Check sheet for the modelled part. Datum: model origin and axes. Units: mm. A direction names the side the tool comes from. Give positions to 0.01 mm unless a question says otherwise; leave off trailing zeros. Write each loop counter-clockwise with the first axis right and the second up, starting at its lowest first coordinate (ties: lowest second). Pieces come first, ordered by that corner, then holes. Notation, with made-up numbers: M 46,84 L 51,84 A23 cw 51,123 Z; hole C 29.5,-9 d2. An arc over 180 degrees is marked long. One line per item, written item: value. Start each with the question number.
from build123d import *

# Parameters (mm, degrees)
BOSS_EXTRUDE1_DEPTH        = 9
BOSS_EXTRUDE2_DEPTH        = 6
BOSS_EXTRUDE3_DEPTH        = 15
BOSS_EXTRUDE3_DEPTH_BACK   = 85
BOSS_EXTRUDE4_DEPTH        = 15
BOSS_EXTRUDE4_DEPTH_BACK   = 35
CUT_EXTRUDE1_DEPTH         = 10
CUT_EXTRUDE2_DEPTH         = 10
BOSS_EXTRUDE6_DEPTH        = 15
BOSS_EXTRUDE6_DEPTH_BACK   = 85
SKETCH1_6_R                = 25
F_25_0_25_DIAMETER_HOLE1_D = 25


with BuildPart() as part:
    # Sketch1 → Boss-Extrude1 (new, symmetric)
    with BuildSketch(Plane.XY):
        with BuildLine():
            Line((-48, 100), (-34, 100))
            ThreePointArc((-34, 100), (0, 66), (34, 100))
            Line((34, 100), (48, 100))
            ThreePointArc((48, 100), (0, 52), (-48, 100))
        make_face()
    extrude(amount=BOSS_EXTRUDE1_DEPTH, both=True)

    # Sketch1<3> → Boss-Extrude2 (add, symmetric)
    with BuildSketch(Plane.XY):
        with BuildLine():
            ThreePointArc((15, 54.403947539), (0, 52), (-15, 54.403947539))
            Line((-15, 54.403947539), (-15, 20))
            ThreePointArc((-15, 20), (0, 25), (15, 20))
            Line((15, 20), (15, 54.403947539))
        make_face()
    extrude(amount=BOSS_EXTRUDE2_DEPTH, both=True)

    # Sketch1<4> → Boss-Extrude3 (add, two sides: drawn at the far end of the back side and taken through both)
    with BuildSketch(Plane.XY.offset(-BOSS_EXTRUDE3_DEPTH_BACK)):
        with BuildLine():
            Line((-15.340741737, -2.588190451), (-25, 0))
            ThreePointArc((-25, 0), (-23.452260867, -8.659760979), (-19.000683183, -16.247277882))
            Line((-19.000683183, -16.247277882), (-15.340741737, -2.588190451))
        make_face()
        with BuildLine():
            ThreePointArc((19.000683183, -16.247277882), (23.452260867, -8.659760979), (25, 0))
            Line((25, 0), (15.340741737, -2.588190451))
            Line((15.340741737, -2.588190451), (19.000683183, -16.247277882))
        make_face()
        with BuildLine():
            ThreePointArc((15, 20), (0, 25), (-15, 20))
            ThreePointArc((-15, 20), (-22.360679775, 11.180339887), (-25, 0))
            Line((-25, 0), (-15.340741737, -2.588190451))
            Line((-15.340741737, -2.588190451), (-19.000683183, -16.247277882))
            ThreePointArc((-19.000683183, -16.247277882), (0, -25), (19.000683183, -16.247277882))
            Line((19.000683183, -16.247277882), (15.340741737, -2.588190451))
            Line((15.340741737, -2.588190451), (25, 0))
            ThreePointArc((25, 0), (22.360679775, 11.180339887), (15, 20))
        make_face()
    extrude(amount=BOSS_EXTRUDE3_DEPTH + BOSS_EXTRUDE3_DEPTH_BACK)

    # Sketch1<5> → Boss-Extrude4 (add, two sides: drawn at the far end of the back side and taken through both)
    with BuildSketch(Plane.XY.offset(-BOSS_EXTRUDE4_DEPTH_BACK)):
        with BuildLine():
            ThreePointArc((-19.000683183, -16.247277882), (-23.452260867, -8.659760979), (-25, 0))
            Line((-25, 0), (-42.599695067, -65.682956188))
            Line((-42.599695067, -65.682956188), (-32.940436804, -68.271146639))
            Line((-32.940436804, -68.271146639), (-19.000683183, -16.247277882))
        make_face()
        with BuildLine():
            Line((42.599695067, -65.682956188), (25, 0))
            ThreePointArc((25, 0), (23.452260867, -8.659760979), (19.000683183, -16.247277882))
            Line((19.000683183, -16.247277882), (32.940436804, -68.271146639))
            Line((32.940436804, -68.271146639), (42.599695067, -65.682956188))
        make_face()
    extrude(amount=BOSS_EXTRUDE4_DEPTH + BOSS_EXTRUDE4_DEPTH_BACK)

    # Sketch3 → Cut-Extrude1 (cut)
    with BuildSketch(Plane(origin=(-23.325317547, 6.25, 0), x_dir=(0, 0, 1), z_dir=(-0.9659258262890681, 0.2588190451025213, 0))):
        with BuildLine():
            Line((-14.115045046, -64.546449271), (-35, -6.470476128))
            Line((-35, -6.470476128), (-35, -74.470476128))
            Line((-35, -74.470476128), (1.18e-07, -74.470476128))
            ThreePointArc((1.18e-07, -74.470476128), (-8.627293932, -71.741164756), (-14.115045046, -64.546449271))
        make_face()
        with BuildLine():
            Line((15, -74.470476128), (15, -59.470476128))
            ThreePointArc((15, -59.470476128), (10.60660176, -70.077077804), (1.18e-07, -74.470476128))
            Line((1.18e-07, -74.470476128), (15, -74.470476128))
        make_face()
        with BuildLine():
            Line((-6, -40.470476128), (-6, -59.470476128))
            ThreePointArc((-6, -59.470476128), (0, -65.470476128), (6, -59.470476128))
            Line((6, -59.470476128), (6, -40.470476128))
            ThreePointArc((6, -40.470476128), (0, -34.470476128), (-6, -40.470476128))
        make_face()
    extrude(amount=-CUT_EXTRUDE1_DEPTH, mode=Mode.SUBTRACT)

    # Sketch4 → Cut-Extrude2 (cut)
    with BuildSketch(Plane(origin=(23.325317547, 6.25, 0), x_dir=(0, 0, -1), z_dir=(0.9659258262890681, 0.2588190451025213, 0))):
        with BuildLine():
            Line((35, -74.470476128), (35, -6.470476128))
            Line((35, -6.470476128), (13.986332308, -64.572126035))
            ThreePointArc((13.986332308, -64.572126035), (8.496673309, -71.749009188), (-0.119452585, -74.470476128))
            Line((-0.119452585, -74.470476128), (35, -74.470476128))
        make_face()
        with BuildLine():
            ThreePointArc((-0.119452585, -74.470476128), (-10.03562817, -70.725229004), (-15, -61.359737742))
            Line((-15, -61.359737742), (-15, -74.470476128))
            Line((-15, -74.470476128), (-0.119452585, -74.470476128))
        make_face()
        with BuildLine():
            Line((-5.999881425, -40.432754995), (-6.119334038, -59.432754995))
            ThreePointArc((-6.119334038, -59.432754995), (-0.157173745, -65.470357553), (5.880428813, -59.50819726))
            Line((5.880428813, -59.50819726), (5.999881425, -40.50819726))
            ThreePointArc((5.999881425, -40.50819726), (0.037721132, -34.470594702), (-5.999881425, -40.432754995))
        make_face()
    extrude(amount=-CUT_EXTRUDE2_DEPTH, mode=Mode.SUBTRACT)

    # Sketch1<6> → Boss-Extrude6 (add, two sides: drawn at the far end of the back side and taken through both)
    with BuildSketch(Plane.XY.offset(-BOSS_EXTRUDE6_DEPTH_BACK)):
        Circle(SKETCH1_6_R)
    extrude(amount=BOSS_EXTRUDE6_DEPTH + BOSS_EXTRUDE6_DEPTH_BACK)

    # Ø25.0 (25) Diameter Hole1 (through all)
    with Locations(Plane(origin=(0, 0, -85), x_dir=(-1, 0, 0), z_dir=(0, 0, -1))):
        with Locations((0, 0)):
            Hole(F_25_0_25_DIAMETER_HOLE1_D / 2)


solid = part.part
1) Cross-section at B-B (y = 5.5). Record the boundary of the cut face in (x, z).
2) Tool access check on faces 4 (the flat face through (-31.72, -25.08, -4.79)), 5 (the cylindrical face through (-27.49, -28.32, 0.13)), 6 (the flat face through (0.7, 65.7, 9)), 7 (the flat face through (15, 37, 0)). Record the directions out of +Z, -Z, +X, -X, +Y, -Y that give a thin tool (end or side, any length) a straight path to the whole face; none if there is none.
3) Cross-section at A-A (x = 0). Record the boundary of the cut face in (y, z), plus the area to 3 significant figures.
4) Cross-section at D-D (y = 28). Record the boundary of the cut face in (x, z).
5) Material ranges on L1, parallel to Z at x = 20.5, y = -14.5; L2, parallel to X at y = -2, z = -59; L3, parallel to Z at x = -30, y = 63.5, recorded low to high. Write a range as from..to.
6) Gauge pin test, flat ends, axial feed: pin 1 (15 mm diameter, centred on x = 0, y = 0, fed in from -Z); pin 2 (13 mm diameter, centred on y = 40.5, z = -2, fed in from -X); pin 3 (5 mm diameter, centred on x = -10, z = -37.5, fed in from +Y); pin 4 (9 mm diameter, centred on x = 5, y = 39.5, fed in from -Z). Record the tip position at first contact, or that the pin passes through.
7) Cross-section at C-C (z = -23.5). Record the boundary of the cut face in (x, y).
8) Draft check along Z on faces 1 (the flat face through (-32, -43, 6)), 2 (the flat face through (31.968, -26.003, -4.794)), 3 (the flat face through (0, 37, -6)). Enter one of: released by +Z, released by -Z, zero draft, split by the parting line, or undercut.
Data:
1. outline: M -24.39,-85 L -11.22,-85 L -11.22,15 L -24.39,15 Z; M 11.22,-85 L 24.39,-85 L 24.39,15 L 11.22,15 Z
2. face 4: +Z, -Z, -X
2. face 5: -X
2. face 6: +Z, +X, -X, +Y
2. face 7: +Z, -Z, +X
3. outline: M -25,-85 L -12.5,-85 L -12.5,15 L -25,15 Z; M 12.5,-85 L 25,-85 L 25,-6 L 52,-6 L 52,-9 L 66,-9 L 66,9 L 52,9 L 52,6 L 25,6 L 25,15 L 12.5,15 Z
3. area: 3,080 mm2
4. outline: M -15,-6 L 15,-6 L 15,6 L -15,6 Z
5. L1: z = -30.36..15
5. L2: x = -24.92..-12.34, 12.34..24.92
5. L3: z = -9..9
6. pin 1: passes through
6. pin 2: stops at x = -15
6. pin 3: stops at y = 23.85
6. pin 4: stops at z = -6
7. outline: M -33.28,-30.89 L -23.62,-33.48 L -19,-16.25 A25 ccw 19,-16.25 L 23.57,-33.3 L 33.23,-30.71 L 25,0 A25 ccw -25,0 Z; hole C 0,0 d25
8. face 1: undercut
8. face 2: zero draft
8. face 3: released by -Z
